Can you work these out from the model? Positions are in its coordinate system, mm. Face numbers are marked on the shaded views. A direction names the side the tool comes from. Round coordinates to 2 decimals unless told otherwise and drop trailing zeros. Loops run counter-clockwise (first coordinate to the right, second up) from the corner with the lowest first, then second, coordinate; pieces in that order, holes last. Notation, with made-up numbers: (21, 16.25) - (56, 16.25) arc R38 ccw to (56, 54.25) - close; hole circle Ø2 at (85.5, -12). An arc over 180 degrees is marked (long way). Answer as CSV lines item,"result".
```python
from build123d import *

# Parameters (mm, degrees)
SKETCH1_W           = 45
SKETCH1_H           = 15
SKETCH1_W_2         = 5
SKETCH1_H_2         = 5
BOSS_EXTRUDE1_DEPTH = 20
SKETCH2_W           = 15
SKETCH2_H           = 15
CUT_EXTRUDE1_DEPTH  = 20
SKETCH3_R           = 1.65
CUT_EXTRUDE2_DEPTH  = 10
CHAMFER2_SIZE       = 1
CHAMFER3_SIZE       = 1


with BuildPart() as part:
    # Sketch1 → Boss-Extrude1 (new body)
    with BuildSketch(Plane(origin=(0, 0, 0), x_dir=(1, 0, 0), z_dir=(0, 1, 0))):
        with Locations((22.5, 7.5)):
            Rectangle(SKETCH1_W, SKETCH1_H)
        with Locations((22.5, 7.5)):
            Rectangle(SKETCH1_W_2, SKETCH1_H_2, mode=Mode.SUBTRACT)
    extrude(amount=BOSS_EXTRUDE1_DEPTH)

    # Sketch2 → Cut-Extrude1 (cut)
    with BuildSketch(Plane.XY):
        with Locations((22.5, 12.5)):
            Rectangle(SKETCH2_W, SKETCH2_H)
    extrude(amount=-CUT_EXTRUDE1_DEPTH, mode=Mode.SUBTRACT)

    # Sketch3 → Cut-Extrude2 (cut)
    with BuildSketch(Plane(origin=(0, 20, 0), x_dir=(1, 0, 0), z_dir=(0, 1, 0))):
        with Locations(Location((37.5, 7.5, 0), (0, 0, 270))):
            Circle(SKETCH3_R)
        with Locations(Location((7.5, 7.5, 0), (0, 0, 270))):
            Circle(SKETCH3_R)
    extrude(amount=-CUT_EXTRUDE2_DEPTH, mode=Mode.SUBTRACT)

    # Chamfer2
    chamfer2_edges = [part.edges().sort_by_distance(p)[0] for p in [
        (45, 20, -7.5),
        (20, 0, -7.5),
        (22.5, 0, -5),
        (25, 0, -7.5),
        (22.5, 0, -10),
        (37.5, 20, -15),
        (7.5, 20, -15),
        (37.5, 20, 0),
        (30, 20, -7.5),
        (15, 20, -7.5),
        (0, 20, -7.5),
        (22.5, 0, -15),
        (45, 0, -7.5),
        (37.5, 20, -9.15),
        (22.5, 0, 0),
        (7.5, 20, -9.15),
        (0, 0, -7.5),
        (7.5, 20, 0),
    ]]
    chamfer(chamfer2_edges, length=CHAMFER2_SIZE)

    # Chamfer3
    chamfer3_edges = [part.edges().sort_by_distance(p)[0] for p in [
        (30, 12, -15),
        (15, 5, -7.5),
        (22.5, 5, -15),
        (30, 5, -7.5),
        (22.5, 5, 0),
        (30, 12, 0),
        (45, 10, -15),
        (45, 10, 0),
        (15, 12, 0),
        (0, 10, 0),
        (15, 12, -15),
        (0, 10, -15),
    ]]
    chamfer(chamfer3_edges, length=CHAMFER3_SIZE)


solid = part.part
```
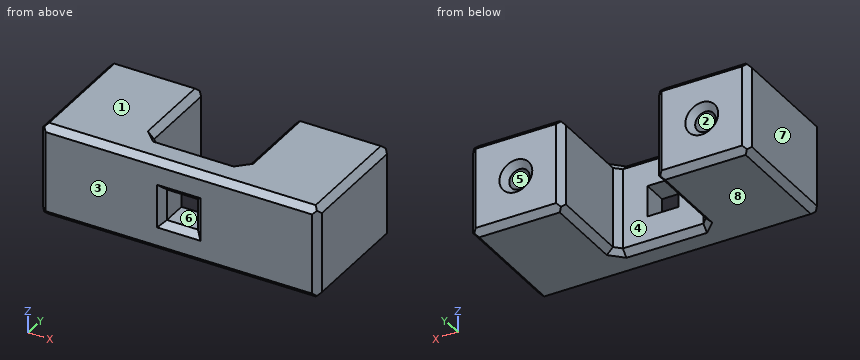
Q1. Imagine slicing it at A-A (y = 16.25). Write out the boundary of the cut face in (x, z), then the cut area to 3 significant figures.
Checks:
outline,"(0, -14) - (1, -15) - (14, -15) - (15, -14) - (15, -1) - (14, 0) - (1, 0) - (0, -1) - close; (30, -14) - (31, -15) - (44, -15) - (45, -14) - (45, -1) - (44, 0) - (31, 0) - (30, -1) - close; hole circle Ø3.3 at (7.5, -7.5); hole circle Ø3.3 at (37.5, -7.5)"
area,"429 mm²"
Q2. Imagine slicing it at D-D (x = 37.5). Write out the boundary of the cut face in (y, z).
Checks:
outline,"(0, -14) - (1, -15) - (19, -15) - (20, -14) - (20, -10.15) - (19, -9.15) - (10, -9.15) - (10, -5.85) - (19, -5.85) - (20, -4.85) - (20, -1) - (19, 0) - (1, 0) - (0, -1) - close"
Q3. I'm going to push flat-ended pins straight in: pin 1 Ø4 at (x, y) = (17, 6.5) entering from +Z; pin 2 Ø1.6 at (x, z) = (37.5, -7) entering from +Y. Where does each tip first touch, or does it pass through?
Checks:
pin 1,"z = -0.5"
pin 2,"y = 10"
Q4. On a 3-axis mill with a long thin cutter (end or side, diameter ignored), from which of +Z, -Z, +X, -X, +Y, -Y can I reach the whole of each face in a straight line? I mean the marked faces 4, 5, 6, 7 and 8. Say none if no direction works.
Checks:
face 4,"+Z, -Z, +Y"
face 5,"+Y"
face 6,"+Y, -Y"
face 7,"+Z, -Z, -X, +Y, -Y"
face 8,"-Z, +X, -X, +Y, -Y"
Q5. Imagine slicing it at C-C (y = 5.5). Write out the boundary of the cut face in (x, z), then the cut area to 3 significant figures.
Checks:
outline,"(0, -14) - (1, -15) - (14.5, -15) - (15.5, -14) - (15.5, -1) - (14.5, 0) - (1, 0) - (0, -1) - close; (29.5, -14) - (30.5, -15) - (44, -15) - (45, -14) - (45, -1) - (44, 0) - (30.5, 0) - (29.5, -1) - close"
area,"461 mm²"
Q6. If I drill on line 1 along X through (y, z) = (17.25, -7.5); line 2 along X through (y, z) = (9.25, -11.75); line 3 along Y through (x, z) = (7.5, -6.25), over which ranges is the centre line in solid material (lowest first)? Write a range as [from, to].
Checks:
line 1,"[0, 5.85], [9.15, 15], [30, 35.85], [39.15, 45]"
line 2,"[0, 15], [30, 45]"
line 3,"[0, 10]"
Q7. We'd pull the mould along Z, two halves only. Please class the marked faces 1, 2 and 3: pulls with the +Z half, pulls with the -Z half, needs draft (parallel to the pull), parting line crosses it, or undercut.
Checks:
face 1,"pulls with the +Z half"
face 2,"undercut"
face 3,"needs draft"
